from build123d import *

# Parameters (mm, degrees)
F1_DEPTH      = 10
F3_DEPTH      = 4
F3_DEPTH_BACK = 14
F4_W          = 10
F4_H          = 10
F5_DEPTH      = 25
F6_T1_DEPTH   = 10
F7_R          = 4
F8_R          = 5
F10_DEPTH     = 60


# Not quite as in the source:
# - a fillet or chamfer that OpenCascade refuses, or shapes differently, is made with other operations: its cross-section is extruded or revolved along the edge and cut away or added
# - a feature names something its author has since deleted; it is built from what else it names


with BuildPart() as f1:
    # F0 (on Front) → F1 (new body)
    with BuildSketch(Plane.XZ):
        with BuildLine():
            ThreePointArc((19.6522871604, -43.3779198274), (22.0356929141, -43.9481357221), (24.344898549, -44.7687077723))
            Line((24.344898549, -44.7687077723), (30.2937477303, -42.2061976958))
            Line((30.2937477303, -42.2061976958), (16.0343749186, -9.1031636608))
            ThreePointArc((16.0343749186, -9.1031636608), (14.7317766807, -2.4774455359), (16.2784975378, 4.0955718405))
            Line((16.2784975378, 4.0955718405), (40, 54))
            Line((40, 54), (31.6958138155, 54))
            Line((31.6958138155, 54), (7.7256415471, 3.5724294089))
            ThreePointArc((7.7256415471, 3.5724294089), (6.6322171557, 2.1826346144), (5.0464276278, 1.4000887411))
            Line((5.0464276278, 1.4000887411), (-16.5758134292, -3.788837771))
            ThreePointArc((-16.5758134292, -3.788837771), (-19.6646678264, -3.268857876), (-21.4317839616, -0.6826055404))
            Line((-21.4317839616, -0.6826055404), (-32.3519113749, 54))
            Line((-32.3519113749, 54), (-40, 54))
            Line((-40, 54), (-27.9160834498, -6.5102868387))
            ThreePointArc((-27.9160834498, -6.5102868387), (-26.9490490541, -9.6402216111), (-25.3648124606, -12.5075969995))
            Line((-25.3648124606, -12.5075969995), (-6.5550611463, -39.5746751924))
            ThreePointArc((-6.5550611463, -39.5746751924), (-4.9098360692, -42.5874005907), (-3.945102256, -45.8817242769))
            Line((-3.945102256, -45.8817242769), (3.8871387568, -40.2303608977))
            Line((3.8871387568, -40.2303608977), (-12.4880276922, -17.5359698901))
            ThreePointArc((-12.4880276922, -17.5359698901), (-12.8770477363, -13.5212266501), (-9.5721086698, -11.2088950032))
            Line((-9.5721086698, -11.2088950032), (5.2830699548, -9.987289736))
            ThreePointArc((5.2830699548, -9.987289736), (7.6708908871, -10.5450664651), (9.284566981, -12.3913744428))
            Line((9.284566981, -12.3913744428), (20.6643672802, -38.8095010734))
            ThreePointArc((20.6643672802, -38.8095010734), (20.8960138101, -41.2571363473), (19.6522871604, -43.3779198274))
        make_face()
        with BuildLine():
            Line((-4.3718418374, -54.4194170272), (-2.8750095458, -56.4938812719))
            Line((-2.8750095458, -56.4938812719), (24.344898549, -44.7687077723))
            ThreePointArc((24.344898549, -44.7687077723), (22.0356929141, -43.9481357221), (19.6522871604, -43.3779198274))
            ThreePointArc((19.6522871604, -43.3779198274), (18.4554525804, -44.1141232898), (17.0778668556, -44.3910097661))
            Line((17.0778668556, -44.3910097661), (9.1481831441, -44.5638505003))
            ThreePointArc((9.1481831441, -44.5638505003), (8.440161238, -44.5163238476), (7.7516789791, -44.3444344023))
            ThreePointArc((7.7516789791, -44.3444344023), (0.7998412321, -48.3108696597), (-4.3718418374, -54.4194170272))
        make_face()
        with BuildLine():
            Line((-4.5614236042, -54.156675103), (-4.3718418374, -54.4194170272))
            ThreePointArc((-4.3718418374, -54.4194170272), (0.7998412321, -48.3108696597), (7.7516789791, -44.3444344023))
            ThreePointArc((7.7516789791, -44.3444344023), (6.6734648322, -43.7740983951), (5.81726752, -42.9053319878))
            Line((5.81726752, -42.9053319878), (3.8871387568, -40.2303608977))
            Line((3.8871387568, -40.2303608977), (-3.945102256, -45.8817242769))
            ThreePointArc((-3.945102256, -45.8817242769), (-3.7026448472, -49.2316692283), (-4.1648631271, -52.5584200507))
            Line((-4.1648631271, -52.5584200507), (-4.5614236042, -54.156675103))
        make_face()
        Polygon((30.2937477303, -42.2061976958), (36.6235819074, -56.9008633705), (45.807747954, -52.9447170098), (39.477913777, -38.2500513351), align=None)
        with BuildLine():
            ThreePointArc((24.344898549, -44.7687077723), (31.6655422142, -49.6392162498), (36.6235819074, -56.9008633705))
            Line((36.6235819074, -56.9008633705), (30.2937477303, -42.2061976958))
            Line((30.2937477303, -42.2061976958), (24.344898549, -44.7687077723))
        make_face()
    extrude(amount=F1_DEPTH)

    # F2 (on face) → F3 (join, two sides)
    with BuildSketch(Plane.XZ.offset(10)) as f3_sk:
        with BuildLine():
            Line((45.807747954, -52.9447170098), (39.477913777, -38.2500513351))
            Line((39.477913777, -38.2500513351), (30.2937477303, -42.2061976958))
            Line((30.2937477303, -42.2061976958), (24.721675481, -44.6064083669))
            ThreePointArc((24.721675481, -44.6064083669), (31.9751079214, -49.5289380846), (36.8958559524, -56.7835793441))
            Line((36.8958559524, -56.7835793441), (45.807747954, -52.9447170098))
        make_face()
        with BuildLine():
            Line((36.6235819074, -56.9008633705), (36.8958559524, -56.7835793441))
            ThreePointArc((36.8958559524, -56.7835793441), (31.9751079214, -49.5289380846), (24.721675481, -44.6064083669))
            ThreePointArc((24.721675481, -44.6064083669), (22.3566538827, -43.7354236695), (19.9113834301, -43.1250189536))
            ThreePointArc((19.9113834301, -43.1250189536), (18.6224089936, -44.0440177459), (17.0778668556, -44.3910097661))
            Line((17.0778668556, -44.3910097661), (9.1481831441, -44.5638505003))
            ThreePointArc((9.1481831441, -44.5638505003), (8.2237355637, -44.4761887941), (7.3444115948, -44.177730654))
            ThreePointArc((7.3444115948, -44.177730654), (0.5352155123, -48.1455807465), (-4.5614236042, -54.156675103))
            Line((-4.5614236042, -54.156675103), (-2.8750095458, -56.4938812719))
            Line((-2.8750095458, -56.4938812719), (24.344898549, -44.7687077723))
            ThreePointArc((24.344898549, -44.7687077723), (31.6655422142, -49.6392162498), (36.6235819074, -56.9008633705))
        make_face()
        with BuildLine():
            Line((29.7354573724, -59.867973141), (36.6235819074, -56.9008633705))
            ThreePointArc((36.6235819074, -56.9008633705), (31.6655422142, -49.6392162498), (24.344898549, -44.7687077723))
            Line((24.344898549, -44.7687077723), (-2.8750095458, -56.4938812719))
            Line((-2.8750095458, -56.4938812719), (0.6883118522, -61.4322988045))
            ThreePointArc((0.6883118522, -61.4322988045), (14.6664598558, -50.5224287814), (29.7354573724, -59.867973141))
        make_face()
    extrude(amount=F3_DEPTH)
    extrude(f3_sk.sketch, amount=-F3_DEPTH_BACK)

    # F4 (on face) → F5 (cut)
    with BuildSketch(Plane(origin=(19.4014510262, 0, 8.35731622), x_dir=(0, 1, 0), z_dir=(0.9184166047, 0, 0.3956146361))):
        with Locations((-5, -61.7475227671)):
            Rectangle(F4_W, F4_H)
    extrude(amount=-F5_DEPTH, mode=Mode.SUBTRACT)

    # F6: fillet of radius 5 on 1 edges, made by hand

    # F6_s2 → F6_t1 (join)
    with BuildSketch(Plane.XZ):
        with BuildLine():
            ThreePointArc((28.31567455, -37.6141146724), (31.0593734872, -40.2818434972), (34.8858307536, -40.2281245155))
            Line((34.8858307536, -40.2281245155), (30.2937477303, -42.2061976958))
            Line((30.2937477303, -42.2061976958), (28.31567455, -37.6141146724))
        make_face()
    extrude(amount=F6_T1_DEPTH)

    # F7
    f7_edges = [f1.edges().sort_by_distance(p)[0] for p in [
        (39.477914, -5, -38.250051),
    ]]
    fillet(f7_edges, radius=F7_R)

    # F8
    f8_edges = [f1.edges().sort_by_distance(p)[0] for p in [
        (45.807748, -12, -52.944717),
        (45.807748, 2, -52.944717),
    ]]
    fillet(f8_edges, radius=F8_R)

    # F9 (on face) → F10 (join)
    with BuildSketch(Plane.XZ.offset(10)):
        with BuildLine():
            ThreePointArc((-17.0067008, -11.8202735087), (-18.8974369177, -8.3589640964), (-20.3653347512, -4.6982507964))
            Line((-20.3653347512, -4.6982507964), (-27.9160834498, -6.5102868387))
            ThreePointArc((-27.9160834498, -6.5102868387), (-26.9490490541, -9.6402216111), (-25.3648124606, -12.5075969995))
            Line((-25.3648124606, -12.5075969995), (-17.0067008, -11.8202735087))
        make_face()
        with BuildLine():
            Line((16.2784975378, 4.0955718405), (7.0391568902, 1.8783058544))
            ThreePointArc((7.0391568902, 1.8783058544), (6.2442508473, -4.0206259595), (7.72081337, -9.7868236042))
            Line((7.72081337, -9.7868236042), (16.0343749186, -9.1031636608))
            ThreePointArc((16.0343749186, -9.1031636608), (14.7317766807, -2.4774455359), (16.2784975378, 4.0955718405))
        make_face()
    extrude(amount=F10_DEPTH)


solid = f1.part
Read the model definition and answer for the solid it produces. Units are mm, in the model's axes. A direction names the side the tool comes from. Give positions to 0.01 mm unless a question says otherwise; leave off trailing zeros. Write each loop counter-clockwise with the first axis right and the second up, starting at its lowest first coordinate (ties: lowest second). Pieces come first, ordered by that corner, then holes. Notation, with made-up numbers: (-0.75, 20.25) - (44.25, 20.25) arc R17 cw to (44.25, 33.25) - close; hole circle Ø9 at (-8, 52.25). An arc over 180 degrees is marked (long way). Use CSV: the item, a comma, the result in double quotes. Start each with the question number.
(1) For faces 4 (the flat face through (32.27, -5.07, -47.89)), 5 (the flat face through (-5.613, -4.93, -1.158)), 6 (the flat face through (-24.088, -39.58, -5.592)), determine the directions among +Z, -Z, +X, -X, +Y, -Y from which every point of the face is accessible in a straight line to the end or side of a thin tool.
(2) Find section C-C (z = -32.5). Give the vertices of the cut face in (x, y).
(3) Given P1, Ø5, axis at y = -10.5, z = 4.5, coming from the -X side; P2, Ø1.5, axis at x = 23.5, z = -32, coming from the +Y side; P3, Ø1.5, axis at x = -20, y = -41, coming from the +Z side; P4, Ø2, axis at y = -12.5, z = 8, coming from the -X side, each flat-ended and moving along its own axis, determine where each tip first touches the part or whether it passes through.
(4) Find section B-B (x = 2). Give the vertices of the cut face in (y, z).
(5) Find section D-D (x = -19). Give the vertices of the cut face in (y, z), plus the area to 3 significant figures.
(6) Determine the mould class of faces 1 (the flat face through (11.72, -39.58, 3)), 2 (the flat face through (27.973, -4.93, 28.698)), 3 (the cylindrical face through (6.24, -39.58, -3.94)) for opening direction X: +X half, -X half, draft (parallel to the pull), parting line (faces both ways), or undercut.
(7) Find section A-A (y = -57). Give the vertices of the cut face in (x, z), plus the area to 3 significant figures.
(8) Consider line 1 along Y through (x, z) = (38.5, -53.5); line 2 along Y through (x, z) = (26.5, 39); line 3 along Z through (x, y) = (2, -5). Determine where each line is inside the solid, lowest interval first.
Findings below:
1,face 4,"-Z, +X"
1,face 5,"+Z, +Y, -Y"
1,face 6,"+Z, -X, -Y"
2,outline,"(-11.47, -10) - (-1.69, -10) - (-1.69, 0) - (-11.47, 0) - close; (17.95, -10) - (26.11, -10) - (26.11, 0) - (17.95, 0) - close"
3,P1,"x = -30.6"
3,P2,"y = 0"
3,P3,"z = -4.7"
3,P4,"through"
4,outline,"(-14, -58.38) - (4, -58.38) - (4, -47.01) - (0, -47.01) - (0, -37.61) - (-10, -37.61) - (-10, -47.01) - (-14, -47.01) - close; (-10, -10.26) - (0, -10.26) - (0, 0.67) - (-10, 0.67) - close"
5,outline,"(-70, -11.98) - (-10, -11.98) - (-10, -21.67) - (0, -21.67) - (0, -3.61) - (-10, -3.61) - (-10, -8.14) - (-70, -8.14) - close"
5,area,"411 mm2"
6,face 1,"-X half"
6,face 2,"+X half"
6,face 3,"undercut"
7,outline,"(-27.92, -6.51) arc R16 ccw to (-25.36, -12.51) - (-17.01, -11.82) arc R33.27 cw to (-20.37, -4.7) - close; (7.04, 1.88) arc R15.57 ccw to (7.72, -9.79) - (16.03, -9.1) arc R16 cw to (16.28, 4.1) - close"
7,area,"162 mm2"
8,line 1,"-14 to -10, 0 to 4"
8,line 2,"-10 to 0"
8,line 3,"-58.38 to -37.61, -10.26 to 0.67"
